Check sheet for the drawn part. Datum: minimum x, y, z corner. Units: mm. A direction names the side the tool comes from. Give positions to 0.01 mm unless a question says otherwise; leave off trailing zeros. Loops run counter-clockwise (first coordinate to the right, second up) from the corner with the lowest first, then second, coordinate; pieces in that order, holes last.
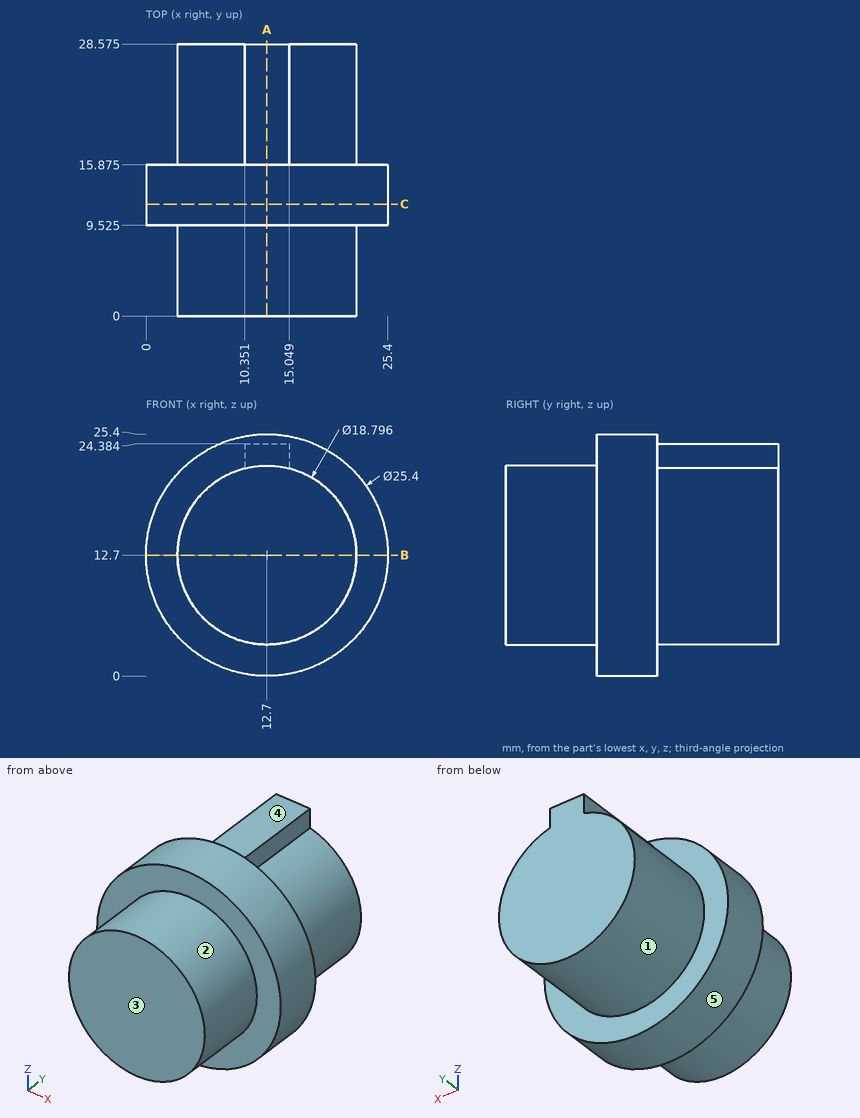
1) Depth check by flat-ended pin: P1, Ø8, axis at x = 6.5, y = 5, coming from the -Z side; P2, Ø2, axis at x = 16.5, y = 12.5, coming from the -Z side; P3, Ø5, axis at x = 20, y = 6, coming from the +Z side. Enter the tip coordinate at first touch or a pass-through.
2) Tool access check on the marked faces 1, 2, 3, 4 and 5. Record the directions out of +Z, -Z, +X, -X, +Y, -Y that give a thin tool (end or side, any length) a straight path to the whole face; none if there is none.
3) Sectioned sample at C-C on y = 11.75. Enter the section's corners in (x, z), plus the area to 3 significant figures.
4) Scan lines: line 1 along X through (y, z) = (15.5, 12.5); line 2 along Y through (x, z) = (2, 8) (1 decimal); line 3 along Z through (x, y) = (16.25, 27.25). Record each from-to range of solid material in increasing order.
5) Sectioned sample at A-A on x = 12.7. Enter the section's corners in (y, z) (1 decimal), plus the area to 3 significant figures.
6) Sectioned sample at B-B on z = 12.7. Enter the section's corners in (x, y) (1 decimal).
Determined:
1. P1: stops at z = 3.56
1. P2: stops at z = 0.31
1. P3: stops at z = 20.78
2. face 1: +Y
2. face 2: -Y
2. face 3: +Z, -Z, +X, -X, -Y
2. face 4: +Z, +X, -X, +Y
2. face 5: +Y, -Y
3. outline: circle Ø25.4 at (12.7, 12.7)
3. area: 507 mm2
4. line 1: x = 0 to 25.4
4. line 2: y = 9.5 to 15.9
4. line 3: z = 4 to 21.4
5. outline: (0, 3.3) - (9.5, 3.3) - (9.5, 0) - (15.9, 0) - (15.9, 3.3) - (28.6, 3.3) - (28.6, 24.4) - (15.9, 24.4) - (15.9, 25.4) - (9.5, 25.4) - (9.5, 22.1) - (0, 22.1) - close
5. area: 608 mm2
6. outline: (0, 9.5) - (3.3, 9.5) - (3.3, 0) - (22.1, 0) - (22.1, 9.5) - (25.4, 9.5) - (25.4, 15.9) - (22.1, 15.9) - (22.1, 28.6) - (3.3, 28.6) - (3.3, 15.9) - (0, 15.9) - close
